Design review of the part built by this model. Coordinates are the model's own, in mm. A direction names the side the tool comes from. Round coordinates to 2 decimals unless told otherwise and drop trailing zeros. Write each loop counter-clockwise with the first axis right and the second up, starting at its lowest first coordinate (ties: lowest second). Pieces come first, ordered by that corner, then holes. Notation, with made-up numbers: M -26.75,87 L -4.75,87 A28 ccw -4.75,119 Z; hole C 76.5,55.25 d6. An arc over 180 degrees is marked long. One line per question, with ' | ' between items. Start each with the question number.
Item 1: Add section C-C, the plane x = -13.5. State the section outline as (y, z) points.
Item 2: Insertion check: pin 1 Ø1.5 at (x, z) = (-55, 3) entering from +Y; pin 2 Ø2.5 at (y, z) = (-48.5, 2.5) entering from -X; pin 3 Ø2.5 at (x, z) = (-56, 2) entering from -Y. Each pin has a flat end and moves straight along its axis. Give the tip position at first contact, or say it passes through.
Item 3: Machinability: for faces 4 (the face through (-27.84, 47, 3)), 5 (the face through (-52.84, -15, 3)), 6 (the face through (-52.84, -102, 3)), which of the approach directions +Z, -Z, +X, -X, +Y, -Y give a long, thin tool a straight path to every point of the face, cutting with its end or side? Answer none if there is none.
Item 4: Add section B-B, the plane y = -73.5. State the section outline as (x, z) points.
Item 5: Draft analysis for pull direction Y (two halves, no side actions). For faces 1 (the face through (-52.84, -45, 3)), 2 (the face through (-55, -97.727, 3)), 3 (the face through (-50, 44.773, 3)), state which applies: released by +Y, released by -Y, zero draft, split by the parting line, or undercut.
Item 6: For L1, parallel to Y at x = -54, z = 0.95; L2, parallel to X at y = -69.5, z = 3.05; L3, parallel to Y at x = -52.5, z = 4.7, list the stretches that pass through material, from the lowest coordinate up.
```python
from build123d import *

# Parameters (mm, degrees)
ESQUISSE1_W             = 50
ESQUISSE1_H             = 155
BOSS_EXTRU_1_DEPTH      = 5
ESQUISSE4_W             = 5
ESQUISSE4_H             = 15
ESQUISSE4_H_2           = 7.5
ESQUISSE4_W_2           = 10
ESQUISSE4_H_3           = 5
ENL_V_MAT_EXTRU_4_DEPTH = 5
ESQUISSE7_W             = 10
ESQUISSE7_H             = 5
ENL_V_MAT_EXTRU_5_DEPTH = 5
ESQUISSE8_W             = 5
ESQUISSE8_H             = 7.5
ENL_V_MAT_EXTRU_6_DEPTH = 5


with BuildPart() as part:
    # Esquisse1 → Boss.-Extru.1 (new body)
    with BuildSketch(Plane.XY):
        with Locations((-32.839977645, -27.727272727)):
            Rectangle(ESQUISSE1_W, ESQUISSE1_H)
    extrude(amount=BOSS_EXTRU_1_DEPTH)

    # Esquisse4 → Enlèv. mat.-Extru.4 (cut)
    with BuildSketch(Plane.XY.offset(5)):
        with Locations((-55.339977645, 14.772727273)):
            Rectangle(ESQUISSE4_W, ESQUISSE4_H)
        with Locations((-55.339977645, -15.227272727)):
            Rectangle(ESQUISSE4_W, ESQUISSE4_H)
        with Locations((-55.339977645, -45.227272727)):
            Rectangle(ESQUISSE4_W, ESQUISSE4_H)
        with Locations((-55.339977645, -75.227272727)):
            Rectangle(ESQUISSE4_W, ESQUISSE4_H)
        with Locations((-55.339977645, -101.477272727)):
            Rectangle(ESQUISSE4_W, ESQUISSE4_H_2)
        with Locations((-32.839977645, 47.272727273)):
            Rectangle(ESQUISSE4_W_2, ESQUISSE4_H_3)
        with Locations((-12.839977645, 47.272727273)):
            Rectangle(ESQUISSE4_W_2, ESQUISSE4_H_3)
    extrude(amount=-ENL_V_MAT_EXTRU_4_DEPTH, mode=Mode.SUBTRACT)

    # Esquisse7 → Enlèv. mat.-Extru.5 (cut)
    with BuildSketch(Plane.XY.offset(5)):
        with Locations((-52.839977645, 47.272727273)):
            Rectangle(ESQUISSE7_W, ESQUISSE7_H)
    extrude(amount=-ENL_V_MAT_EXTRU_5_DEPTH, mode=Mode.SUBTRACT)

    # Esquisse8 → Enlèv. mat.-Extru.6 (cut)
    with BuildSketch(Plane.XY.offset(5)):
        with Locations((-55.339977645, 41.022727273)):
            Rectangle(ESQUISSE8_W, ESQUISSE8_H)
    extrude(amount=-ENL_V_MAT_EXTRU_6_DEPTH, mode=Mode.SUBTRACT)


solid = part.part
```
Computed values:
1) outline: M -105.23,0 L 44.77,0 L 44.77,5 L -105.23,5 Z
2) pin 1: stops at y = 37.27 | pin 2: stops at x = -52.84 | pin 3: stops at y = -97.73
3) face 4: +Z, -Z, +Y | face 5: +Z, -Z, -X | face 6: +Z, -Z, -X, -Y
4) outline: M -52.84,0 L -7.84,0 L -7.84,5 L -52.84,5 Z
5) face 1: undercut | face 2: released by -Y | face 3: released by +Y
6) L1: y = -97.73 to -82.73, -67.73 to -52.73, -37.73 to -22.73, -7.73 to 7.27, 22.27 to 37.27 | L2: x = -52.84 to -7.84 | L3: y = -105.23 to 44.77
